from build123d import *

# Parameters (mm, degrees)
BOSS_EXTRUDE1_DEPTH = 28.668


with BuildPart() as part:
    # Sketch1 → Boss-Extrude1 (new body)
    with BuildSketch(Plane.XY):
        with BuildLine():
            Line((-15.875, -1.5), (-15.023105626, -1.5))
            ThreePointArc((-15.023105626, -1.5), (-10.9, -0.5), (-6.776894374, -1.5))
            Line((-6.776894374, -1.5), (6.776894374, -1.5))
            ThreePointArc((6.776894374, -1.5), (10.9, -0.5), (15.023105626, -1.5))
            Line((15.023105626, -1.5), (15.875, -1.5))
            Line((15.875, -1.5), (15.875, 1.5))
            Line((15.875, 1.5), (-15.875, 1.5))
            Line((-15.875, 1.5), (-15.875, -1.5))
        make_face()
    extrude(amount=BOSS_EXTRUDE1_DEPTH)


solid = part.part
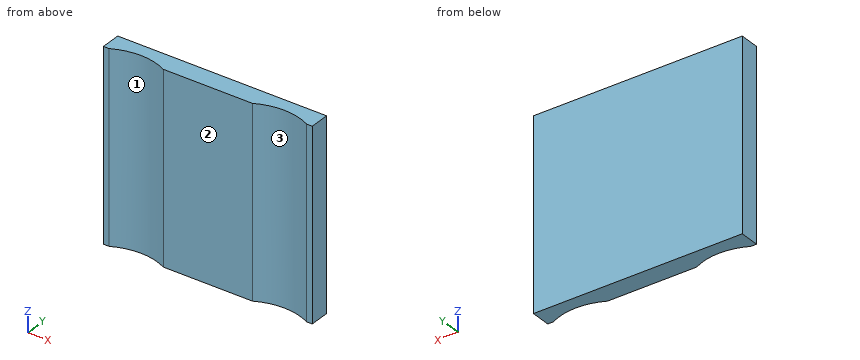
Could you check a few things on this model? Use its own coordinates, in mm. Face numbers are marked on the shaded views. Give positions to 0.01 mm unless a question says otherwise; leave off trailing zeros. Order: outer loops, then holes, each group sorted by start corner. A loop starts at its lowest first (then second) coordinate and runs counter-clockwise, first axis right, second up.
1. Suppose I cut it at B-B (x = 9). List the corners of the cut face in (y, z) for me.
2. Suppose I cut it at A-A (z = 20.75). List the corners of the cut face in (x, y) for me (3 decimals), plus the area to 3 significant figures.
3. We'd pull the mould along X, two halves only. Please class the marked faces 1, 2 and 3: pulls with the +X half, pulls with the -X half, needs draft (parallel to the pull), parting line crosses it, or undercut.
4. Suppose I cut it at C-C (x = -12). List the corners of the cut face in (y, z) for me, plus the area to 3 significant figures.
5. I need wall thicknesses on L1, parallel to X at y = -1.4, z = 22 (3 decimals); L2, parallel to Y at x = -10.5, z = 7.5; L3, parallel to Y at x = 14.5, z = 8.25. Which ranges of each line are inside material? Lowest first, please.
Solved:
1. outline: (-0.7, 0) - (1.5, 0) - (1.5, 28.67) - (-0.7, 28.67) - close
2. outline: (-15.875, -1.5) - (-15.023, -1.5) arc R9 cw to (-6.777, -1.5) - (6.777, -1.5) arc R9 cw to (15.023, -1.5) - (15.875, -1.5) - (15.875, 1.5) - (-15.875, 1.5) - close
2. area: 84.1 mm2
3. face 1: undercut
3. face 2: needs draft
3. face 3: undercut
4. outline: (-0.57, 0) - (1.5, 0) - (1.5, 28.67) - (-0.57, 28.67) - close
4. area: 59.3 mm2
5. L1: x = -15.875 to -14.823, -6.977 to 6.977, 14.823 to 15.875
5. L2: y = -0.51 to 1.5
5. L3: y = -1.25 to 1.5
